```python
from build123d import *

# Parameters (mm, degrees)
F1_DEPTH       = 43
F3_D           = 3.3
F3_CSINK_D     = 6.72
F3_CSINK_ANGLE = 90
F4_SIZE2       = 3
F4_SIZE        = 30
F6_DEPTH       = 1


with BuildPart() as f1:
    # F0 (on Front) → F1 (new body)
    with BuildSketch(Plane.XZ):
        Polygon((0, 74), (0, 0), (105, 0), (105, 4), (5, 4), (5, 74), align=None)
    extrude(amount=-F1_DEPTH)

    # F3 (through all)
    with Locations(Plane.YZ.offset(5)):
        with Locations((31.5, 34), (11.5, 34)):
            CounterSinkHole(F3_D / 2, F3_CSINK_D / 2, counter_sink_angle=F3_CSINK_ANGLE)

    # F4
    f4_edges = [f1.edges().sort_by_distance(p)[0] for p in [
        (105, 21.5, 0),
    ]]
    f4_side = f1.faces().sort_by_distance((52.5, 21.5, 0))[0]
    chamfer(f4_edges, length=F4_SIZE, length2=F4_SIZE2, reference=f4_side)

    # F5 (on face) → F6 (join)
    with BuildSketch(Plane(origin=(0, 43, 0), x_dir=(-1, 0, 0), z_dir=(0, 1, 0))):
        Polygon((-35, 4), (-5, 4), (-5, 19), align=None)
    extrude(amount=-F6_DEPTH)


solid = f1.part
```
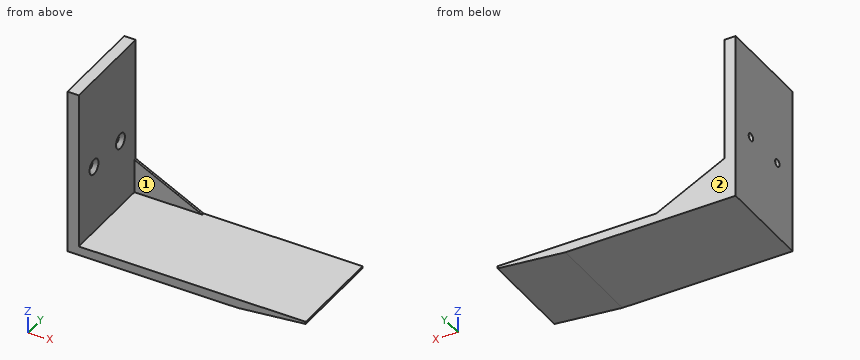
Could you check a few things on this model? Use its own coordinates, in mm. Face numbers are marked on the shaded views. A direction names the side the tool comes from. Round coordinates to 2 decimals unless told otherwise and drop trailing zeros. Loops run counter-clockwise (first coordinate to the right, second up) from the corner with the lowest first, then second, coordinate; pieces in that order, holes last. Notation, with made-up numbers: (-14.75, 29) - (11.25, 29) arc R23 ccw to (11.25, 52) - close; hole circle Ø4 at (-8.5, 56.5). An arc over 180 degrees is marked (long way). Answer as CSV lines item,"result".
1. On a 3-axis mill with a long thin cutter (end or side, diameter ignored), from which of +Z, -Z, +X, -X, +Y, -Y can I reach the whole of each face in a straight line? I mean the marked faces 1 and 2. Say none if no direction works.
Filled in:
face 1,"+Z, +X, -Y"
face 2,"+Z, -Z, +X, -X, +Y"
2. I want a section at A-A on z = 34. List the corners of the cut face in (x, y) for me.
Filled in:
outline,"(0, 0) - (5, 0) - (5, 8.14) - (3.29, 9.85) - (0, 9.85) - close; (0, 13.15) - (3.29, 13.15) - (5, 14.86) - (5, 28.14) - (3.29, 29.85) - (0, 29.85) - close; (0, 33.15) - (3.29, 33.15) - (5, 34.86) - (5, 43) - (0, 43) - close"
3. Please list where these lines run through material, in increasing order: line 1 along Y through (x, z) = (2, 34); line 2 along Z through (x, y) = (1.8, 31.5); line 3 along Z through (x, y) = (20, 24.5). Write a range as [from, to].
Filled in:
line 1,"y = [0, 9.85], [13.15, 29.85], [33.15, 43]"
line 2,"z = [0, 32.35], [35.65, 74]"
line 3,"z = [0, 4]"
4. I want a section at B-B on y = 31.5. List the corners of the cut face in (x, z) for me.
Filled in:
outline,"(0, 0) - (75, 0) - (105, 3) - (105, 4) - (5, 4) - (5, 30.64) - (3.29, 32.35) - (0, 32.35) - close; (0, 35.65) - (3.29, 35.65) - (5, 37.36) - (5, 74) - (0, 74) - close"
5. I want a section at C-C on x = 13. List the corners of the cut face in (y, z) for me, then the cut area to 3 significant figures.
Filled in:
outline,"(0, 0) - (43, 0) - (43, 15) - (42, 15) - (42, 4) - (0, 4) - close"
area,"183 mm^2"
6. For pin 1 Ø13 at (y, z) = (24, 25) entering from +X; pin 2 Ø4 at (y, z) = (31.5, 34) entering from -X; pin 3 Ø21.5 at (x, y) = (37.5, 17) entering from +Z; pin 4 Ø4 at (y, z) = (11.5, 34) entering from +X, each with a flat end and sliding along its axis, tell me the tip position at first contact or that it passes through.
Filled in:
pin 1,"stops at x = 5"
pin 2,"stops at x = 0"
pin 3,"stops at z = 4"
pin 4,"stops at x = 3.64"
7. I want a section at D-D on y = 19.5. List the corners of the cut face in (x, z) for me, then the cut area to 3 significant figures.
Filled in:
outline,"(0, 0) - (75, 0) - (105, 3) - (105, 4) - (5, 4) - (5, 74) - (0, 74) - close"
area,"725 mm^2"
